For this review, take the finished solid that the model builds, in its own axes (mm). Face numbers are marked on the shaded views. A direction names the side the tool comes from. Coordinates: 2 decimals unless noted, no trailing zeros. Write each loop counter-clockwise with the first axis right and the second up, starting at its lowest first coordinate (ties: lowest second). Pieces come first, ordered by that corner, then holes. Notation, with made-up numbers: (-3.75, -27.5) -> (20.25, -27.5) arc R25 ccw to (20.25, -1.5) -> close; hole circle Ø2 at (-24.75, -14.75). An arc over 180 degrees is marked (long way). Put each result on its own line as item: value. Start each with the question number.
Item 1: Consider section D-D on y = 13.5. Give the boundary of the cut face in (x, z), and give its area (3 significant figures).
Item 2: To check wall thickness, follow L1, parallel to X at y = 8, z = 2.75; L2, parallel to Z at x = 14, y = 5; L3, parallel to X at y = -10, z = 2.5. State the ranges of each line that lie inside material, in increasing order.
Item 3: Insertion check: P1, Ø3, axis at x = 52.5, z = -3.5, coming from the +Y side; P2, Ø3, axis at x = -6, y = -11, coming from the +Z side; P3, Ø1, axis at x = -10, z = 3.5, coming from the +Y side. Each pin has a flat end and moves straight along its axis. Give the tip position at first contact, or say it passes through.
Item 4: Consider section C-C on x = 40. Give the boundary of the cut face in (y, z), and give its area (3 significant figures).
Item 5: Consider section A-A on x = -6. Give the boundary of the cut face in (y, z).
Item 6: Consider section B-B on y = 3. Give the boundary of the cut face in (x, z), and give its area (3 significant figures).
Item 7: The part is to be moulded in two halves that separate along Y. For the marked faces 1, 2 and 3, say which applies: +Y half, -Y half, draft (parallel to the pull), parting line (faces both ways), or undercut.
Item 8: For the marked faces 4, 5 and 6, list the 3-axis set-ups (+Z, -Z, +X, -X, +Y, -Y) from which the entire face can be reached by the end or side of a thin tool; tool diameter is ignored.
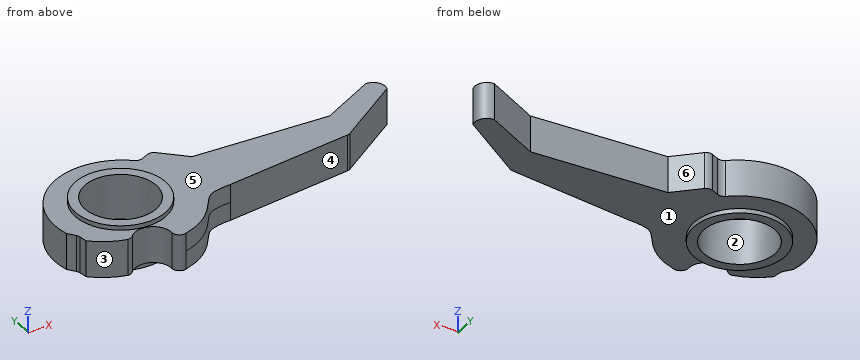
```python
from build123d import *

# Parameters (mm, degrees)
F0_R     = 7.9
F1_DEPTH = 4.02
F2_R     = 10.03
F2_R_2   = 7.9
F3_DEPTH = 5
F4_R     = 1.524


with BuildPart() as f1:
    # F0 (on Top) → F1 (new body, symmetric)
    with BuildSketch(Plane.XY):
        with BuildLine():
            Line((46.1461601803, 4.9444199044), (16.6679395434, 6.772526574))
            Line((16.6679395434, 6.772526574), (10.8789355268, 12.3330182403))
            Line((10.8789355268, 12.3330182403), (7.4512350625, 10.8095955786))
            ThreePointArc((7.4512350625, 10.8095955786), (-10.3629347072, 13.2103242145), (-17.6852336109, -3.2058897622))
            Line((-17.6852336109, -3.2058897622), (-16.1899196828, -5.1818019859))
            Line((-16.1899196828, -5.1818019859), (-15.8845459898, -7.3533461493))
            ThreePointArc((-15.8845459898, -7.3533461493), (-12.6610311769, -9.7318403738), (-8.9288197387, -11.1874777966))
            ThreePointArc((-8.9288197387, -11.1874777966), (-8.17872411, -11.0156404916), (-7.5716043744, -10.5428010492))
            ThreePointArc((-7.5716043744, -10.5428010492), (-3.0198455719, -9.6773974333), (-0.6885354025, -13.6814484455))
            ThreePointArc((-0.6885354025, -13.6814484455), (-0.0064651636, -14.9365604515), (1.3988035828, -15.1929697119))
            add(Edge.make_bspline(
                [(1.3988035828, -15.1929697119), (2.268737628, -14.9110562135), (3.968289553, -14.360236217), (6.0326052215, -13.2728896797), (8.2551576398, -11.498992535), (10.0987298539, -9.2692275408), (11.6138570475, -7.0035918777), (13.3410886509, -5.5985693686), (16.1056359582, -5.3166150456), (17.57795468, -5.2708741645)],
                knots=[0, 0, 0, 0, 0.1403793354, 0.2707223402, 0.413910691, 0.5609255525, 0.7002489917, 0.8244285886, 1, 1, 1, 1], degree=3))
            Line((17.57795468, -5.2708741645), (45.839598026, -2.4268767753))
            Line((45.839598026, -2.4268767753), (60.3782066509, 7.2202376408))
            ThreePointArc((60.3782066509, 7.2202376408), (60.0804354266, 9.6791863318), (57.8765136264, 10.8095955786))
            Line((57.8765136264, 10.8095955786), (46.1461601803, 4.9444199044))
        make_face()
        with Locations((-3.0745326542, 0.769972596)):
            Circle(F0_R, mode=Mode.SUBTRACT)
    extrude(amount=F1_DEPTH, both=True)

    # F2 (on Top) → F3 (join, symmetric)
    with BuildSketch(Plane.XY):
        with Locations((-3.0745326542, 0.769972596)):
            Circle(F2_R)
        with Locations((-3.0745326542, 0.769972596)):
            Circle(F2_R_2, mode=Mode.SUBTRACT)
    extrude(amount=F3_DEPTH, both=True)

    # F4
    f4_edges = [f1.edges().sort_by_distance(p)[0] for p in [
        (-16.18992, -5.181802, 0),
        (7.451235, 10.809596, 0),
        (10.878936, 12.333018, 0),
        (45.839598, -2.426877, 0),
    ]]
    fillet(f4_edges, radius=F4_R)


solid = f1.part
```
Return value:
1. outline: (-9.82, -4.02) -> (3.7, -4.02) -> (3.7, 4.02) -> (-9.82, 4.02) -> close
1. area: 109 mm^2
2. L1: -15.81 to -6.26, 0.11 to 15.39, 52.26 to 60.55
2. L2: -4.02 to 4.02
2. L3: -12.15 to -6.92, -2.44 to 9.47
3. P1: y = 8.87
3. P2: z = 4.02
3. P3: y = 13.66
4. outline: (-3.01, -4.02) -> (5.33, -4.02) -> (5.33, 4.02) -> (-3.01, 4.02) -> close
4. area: 67.1 mm^2
5. outline: (-9.54, -4.02) -> (-8.82, -4.02) -> (-8.82, -5) -> (-6.57, -5) -> (-6.57, 5) -> (-8.82, 5) -> (-8.82, 4.02) -> (-9.54, 4.02) -> close; (8.11, -5) -> (10.36, -5) -> (10.36, -4.02) -> (14.82, -4.02) -> (14.82, 4.02) -> (10.36, 4.02) -> (10.36, 5) -> (8.11, 5) -> close
6. outline: (-17.78, -4.02) -> (-12.85, -4.02) -> (-12.85, -5) -> (-10.65, -5) -> (-10.65, 5) -> (-12.85, 5) -> (-12.85, 4.02) -> (-17.78, 4.02) -> close; (4.5, -5) -> (6.7, -5) -> (6.7, -4.02) -> (54.02, -4.02) -> (54.02, 4.02) -> (6.7, 4.02) -> (6.7, 5) -> (4.5, 5) -> close
6. area: 464 mm^2
7. face 1: draft
7. face 2: undercut
7. face 3: -Y half
8. face 4: +Z, -Z, +X, -Y
8. face 5: +Z
8. face 6: +Z, -Z, +Y
